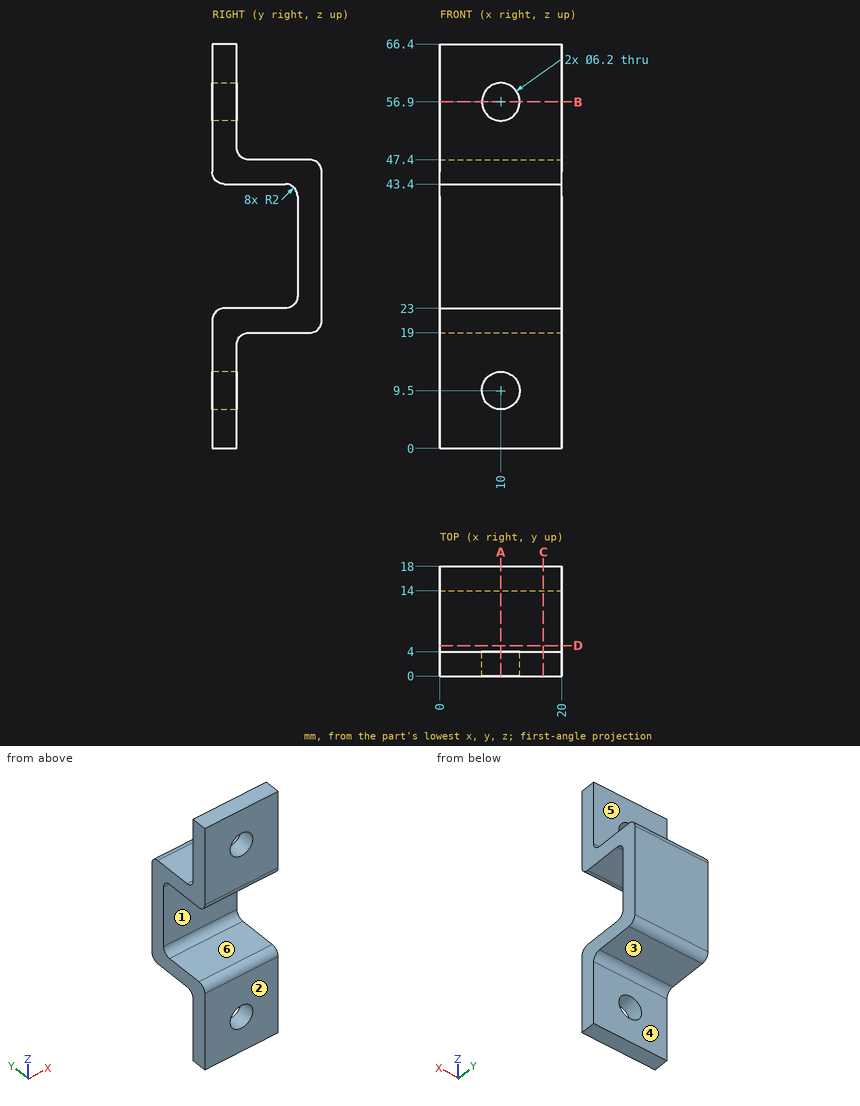
Check sheet for the drawn part. Datum: minimum x, y, z corner. Units: mm. A direction names the side the tool comes from. Give positions to 0.01 mm unless a question says otherwise; leave off trailing zeros. Write each loop counter-clockwise with the first axis right and the second up, starting at its lowest first coordinate (ties: lowest second). Pieces come first, ordered by that corner, then holes.
(1) Cross-section at C-C (x = 17). Enter the section's corners in (y, z).
(2) Mould release check, pull along Z, two halves, no side actions. Record for the marked faces 1, 2 and 3: +Z half, -Z half, draft (parallel to the pull), parting line (faces both ways), or undercut.
(3) Access from +Z, -Z, +X, -X, +Y, -Y to the whole of each face (thin tool, end or side, straight path). Record for the marked faces 4, 5 and 6.
(4) Cross-section at D-D (y = 5). Enter the section's corners in (x, z), plus the area to 3 significant figures.
(5) Cross-section at A-A (x = 10). Enter the section's corners in (y, z).
(6) Material ranges on line 1 (Z direction, x = 18.75, y = 11.75); line 2 (X direction, y = 1.45, z = 56.9); line 3 (Z direction, x = 11.75, y = 3.5), recorded low to high.
(7) Gauge pin test, flat ends, axial feed: pin 1 (8 mm diameter, centred on x = 13.5, y = 9.5, fed in from -Z); pin 2 (5 mm diameter, centred on x = 10.5, y = 9, fed in from +Z); pin 3 (1.5 mm diameter, centred on x = 3, y = 10, fed in from -Z). Record the tip position at first contact, or that the pin passes through.
(8) Cross-section at B-B (z = 56.9). Enter the section's corners in (x, y).
Worked out:
1. outline: (0, 0) - (4, 0) - (4, 17) arc R2 cw to (6, 19) - (16, 19) arc R2 ccw to (18, 21) - (18, 45.4) arc R2 ccw to (16, 47.4) - (6, 47.4) arc R2 cw to (4, 49.4) - (4, 66.4) - (0, 66.4) - (0, 45.4) arc R2 ccw to (2, 43.4) - (12, 43.4) arc R2 cw to (14, 41.4) - (14, 25) arc R2 cw to (12, 23) - (2, 23) arc R2 ccw to (0, 21) - close
2. face 1: undercut
2. face 2: draft
2. face 3: -Z half
3. face 4: -Z, +X, -X, +Y
3. face 5: +Z, +X, -X, +Y
3. face 6: +X, -X, -Y
4. outline: (0, 18.73) - (20, 18.73) - (20, 23) - (0, 23) - close; (0, 43.4) - (20, 43.4) - (20, 47.67) - (0, 47.67) - close
4. area: 171 mm2
5. outline: (0, 0) - (4, 0) - (4, 6.4) - (0, 6.4) - close; (0, 12.6) - (4, 12.6) - (4, 17) arc R2 cw to (6, 19) - (16, 19) arc R2 ccw to (18, 21) - (18, 45.4) arc R2 ccw to (16, 47.4) - (6, 47.4) arc R2 cw to (4, 49.4) - (4, 53.8) - (0, 53.8) - (0, 45.4) arc R2 ccw to (2, 43.4) - (12, 43.4) arc R2 cw to (14, 41.4) - (14, 25) arc R2 cw to (12, 23) - (2, 23) arc R2 ccw to (0, 21) - close; (0, 60) - (4, 60) - (4, 66.4) - (0, 66.4) - close
6. line 1: z = 19 to 23, 43.4 to 47.4
6. line 2: x = 0 to 6.9, 13.1 to 20
6. line 3: z = 0 to 6.94, 12.06 to 23, 43.4 to 54.34, 59.46 to 66.4
7. pin 1: stops at z = 18.94
7. pin 2: stops at z = 47.4
7. pin 3: stops at z = 19
8. outline: (0, 0) - (6.9, 0) - (6.9, 4) - (0, 4) - close; (13.1, 0) - (20, 0) - (20, 4) - (13.1, 4) - close
